Part model, mm, in its own coordinate system. Face numbers are marked on the shaded views. Coordinates: 2 decimals unless noted, no trailing zeros. Order: outer loops, then holes, each group sorted by start corner. A loop starts at its lowest first (then second) coordinate and runs counter-clockwise, first axis right, second up. Notation, with made-up numbers: (27, 83) - (74, 83) arc R22 ccw to (74, 112) - close; hole circle Ø7 at (37.25, 66). An arc over 180 degrees is marked (long way). Use a Markdown table: item, result. Add a question column.
1) Drop flat-ended pins along their axis: P1, Ø0.6, axis at x = 40.5, z = 13.5, coming from the +Y side; P2, Ø2, axis at x = -21, z = -14, coming from the -Y side; P3, Ø13, axis at x = 5.5, z = -0.5, coming from the -Y side; P4, Ø1, axis at x = -4.5, y = 16, coming from the +Z side. Give the stop position or say it passes through.
2) Saw through at D-D on y = 19. List the corners of the cut face in (x, z).
3) Saw through at A-A on x = -69. List the corners of the cut face in (y, z).
4) Two-plate mould, pull along Z, no slides. Class the marked faces 1, 2, 3 and 4: +Z half, -Z half, draft (parallel to the pull), parting line (faces both ways), or undercut.
5) Saw through at B-B on x = 26. List the corners of the cut face in (y, z), then the cut area to 3 significant figures.
6) Saw through at C-C on y = 36. List the corners of the cut face in (x, z).
7) Wall check: L1, parallel to Z at x = 46, y = 7.5; L2, parallel to Y at x = -47, z = 5; L3, parallel to Y at x = 51, z = 14. Give the ranges that are in metal, low to high. Write a range as [from, to].
```python
from build123d import *

# Parameters (mm, degrees)
BOSS_EXTRUDE1_DEPTH = 2
BOSS_EXTRUDE2_DEPTH = 26
BOSS_EXTRUDE3_START = 2
BOSS_EXTRUDE3_DEPTH = 2
CUT_EXTRUDE1_REACH  = 138.664
CUT_EXTRUDE2_DEPTH  = 137.663822213
HOLE1_D             = 1.156713631
HOLE1_DEPTH         = 2
HOLE2_D             = 7.232882037
HOLE2_DEPTH         = 2
FILLET1_R           = 2
FILLET2_R           = 4
FILLET3_R           = 6
FILLET4_R           = 7
FILLET5_R           = 9


with BuildPart() as part:
    # Sketch1 → Boss-Extrude1 (new body)
    with BuildSketch(Plane.XY.offset(-13)):
        with BuildLine():
            Line((38.589514728, 53.714517423), (38.390964743, 54.000002708))
            Line((38.390964743, 54.000002708), (37, 56.000002696))
            Line((37, 56.000002696), (-79, 56.000002696))
            Line((-79, 56.000002696), (-84.797547627, 44.113268525))
            ThreePointArc((-84.797547627, 44.113268525), (-103.30638504, 33.384611029), (-109.961112948, 13.052475123))
            ThreePointArc((-109.961112948, 13.052475123), (-114.714513302, 9.85906483), (-118.822624433, 5.869565217))
            ThreePointArc((-118.822624433, 5.869565217), (-117.511822587, -7.114760135), (-104.611841725, -5.139563921))
            Line((-104.611841725, -5.139563921), (-76.511157838, -5.139563921))
            ThreePointArc((-76.511157838, -5.139563921), (-66.310042494, -8.694638462), (-59.898757812, 0))
            Line((-59.898757812, 0), (59.520798297, 0))
            ThreePointArc((59.520798297, 0), (81.317661031, -7.891849144), (88.119135563, 14.269478708))
            Line((88.119135563, 14.269478708), (68.507754464, 49.131976199))
            Line((68.507754464, 49.131976199), (42.308532947, 53.113281503))
            Line((42.308532947, 53.113281503), (41.5, 54.000002696))
            Line((41.5, 54.000002696), (39.5, 54.000002696))
            ThreePointArc((39.5, 54.000002696), (39.14959506, 53.522905936), (38.589514728, 53.714517423))
        make_face()
    extrude(amount=-BOSS_EXTRUDE1_DEPTH)

    # Sketch2 → Boss-Extrude2 (add)
    with BuildSketch(Plane.XY.offset(-13)):
        Polygon((37, 56.000002696), (38.390964806, 54.000002752), (-79.97546515, 54.000002752), (-79, 56.000002696), align=None)
    extrude(amount=BOSS_EXTRUDE2_DEPTH)

    # Sketch3 → Boss-Extrude3 (add)
    with BuildSketch(Plane.XY.offset(13).offset(BOSS_EXTRUDE3_START)):
        with BuildLine():
            Line((39.500000002, 54.000002689), (41.499999991, 54.000002689))
            Line((41.499999991, 54.000002689), (42.308532938, 53.113281497))
            Line((42.308532938, 53.113281497), (68.507754455, 49.131976193))
            Line((68.507754455, 49.131976193), (88.119135607, 14.269478608))
            ThreePointArc((88.119135607, 14.269478608), (81.317661026, -7.891849269), (59.520798297, 0))
            Line((59.520798297, 0), (-59.898757812, 0))
            ThreePointArc((-59.898757812, 0), (-66.310042494, -8.694638462), (-76.511157838, -5.139563921))
            Line((-76.511157838, -5.139563921), (-104.611841725, -5.139563921))
            ThreePointArc((-104.611841725, -5.139563921), (-117.511822587, -7.114760135), (-118.822624433, 5.869565217))
            ThreePointArc((-118.822624433, 5.869565217), (-114.714513302, 9.85906483), (-109.961112948, 13.052475123))
            ThreePointArc((-109.961112948, 13.052475123), (-103.30638504, 33.384611029), (-84.797547627, 44.113268525))
            Line((-84.797547627, 44.113268525), (-79, 56.000002696))
            Line((-79, 56.000002696), (37, 56.000002696))
            Line((37, 56.000002696), (38.589345234, 53.714761246))
            ThreePointArc((38.589345234, 53.714761246), (39.149453375, 53.522861518), (39.500000002, 54.000002689))
        make_face()
    extrude(amount=-BOSS_EXTRUDE3_DEPTH)

    # Sketch4 → Cut-Extrude1 (cut, up to next)
    with BuildSketch(Plane(origin=(0, 0, -15), x_dir=(-1, 0, 0), z_dir=(0, 0, -1)), mode=Mode.PRIVATE) as cut_extrude1_sk1:
        with BuildLine():
            Line((-37, 14.999963704), (42, 14.999963704))
            ThreePointArc((42, 14.999963704), (48.5, 21.499963704), (42, 27.999963704))
            Line((42, 27.999963704), (-37, 27.999963704))
            ThreePointArc((-37, 27.999963704), (-43.5, 21.499963704), (-37, 14.999963704))
        make_face()
    cut_extrude1_tool1 = extrude(cut_extrude1_sk1.sketch, amount=-CUT_EXTRUDE1_REACH, mode=Mode.PRIVATE) & part.part
    add(cut_extrude1_tool1.solids().sort_by_distance((-2.5, 21.499964, -15))[0], mode=Mode.SUBTRACT)

    # Sketch5 → Cut-Extrude2 (cut, through all)
    with BuildSketch(Plane.XY.offset(15)):
        with BuildLine():
            Line((37, 27.999963704), (-42, 27.999963704))
            ThreePointArc((-42, 27.999963704), (-48.5, 21.499963704), (-42, 14.999963704))
            Line((-42, 14.999963704), (37, 14.999963704))
            ThreePointArc((37, 14.999963704), (43.5, 21.499963704), (37, 27.999963704))
        make_face()
    extrude(amount=-CUT_EXTRUDE2_DEPTH, mode=Mode.SUBTRACT)

    # Hole1
    with Locations(Plane(origin=(0, 0, 13), x_dir=(-1, 0, 0), z_dir=(0, 0, -1))):
        with Locations((-78.000162744, 0)):
            Hole(HOLE1_D / 2, depth=HOLE1_DEPTH)

    # Hole2
    with Locations(Plane.XY.offset(-13)):
        with Locations((-69, 0)):
            Hole(HOLE2_D / 2, depth=HOLE2_DEPTH)

    # Fillet1
    fillet1_edges = [part.edges().sort_by_distance(p)[0] for p in [
        (42.308532947, 53.113281503, -14),
        (42.308532938, 53.113281497, 14),
    ]]
    fillet(fillet1_edges, radius=FILLET1_R)

    # Fillet2
    fillet2_edges = [part.edges().sort_by_distance(p)[0] for p in [
        (-84.797547627, 44.113268525, -14),
        (-84.797547627, 44.113268525, 14),
    ]]
    fillet(fillet2_edges, radius=FILLET2_R)

    # Fillet3
    fillet3_edges = [part.edges().sort_by_distance(p)[0] for p in [
        (-109.961112948, 13.052475123, -14),
        (-109.961112948, 13.052475123, 14),
    ]]
    fillet(fillet3_edges, radius=FILLET3_R)

    # Fillet4
    fillet4_edges = [part.edges().sort_by_distance(p)[0] for p in [
        (-59.898757812, 0, -14),
        (-76.511157838, -5.139563921, -14),
        (-104.611841725, -5.139563921, -14),
        (-104.611841725, -5.139563921, 14),
        (-76.511157838, -5.139563921, 14),
        (-59.898757812, 0, 14),
    ]]
    fillet(fillet4_edges, radius=FILLET4_R)

    # Fillet5
    fillet5_edges = [part.edges().sort_by_distance(p)[0] for p in [
        (59.520798297, 0, -14),
        (59.520798297, 0, 14),
    ]]
    fillet(fillet5_edges, radius=FILLET5_R)


solid = part.part
```
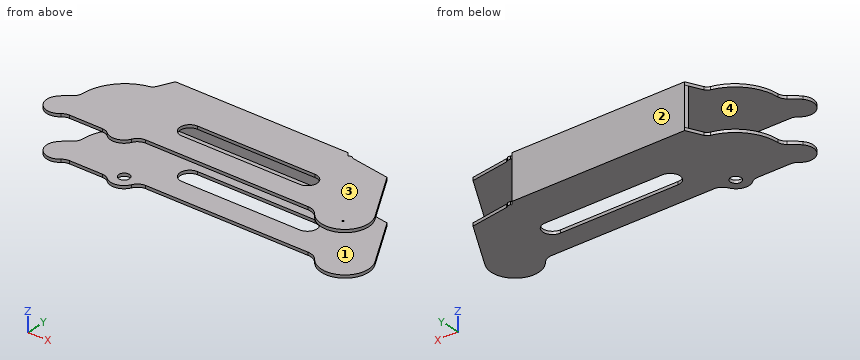
Results are:
| question | item | result |
|---|---|---|
| 1 | P1 | y = 54 |
| 1 | P2 | y = 0 |
| 1 | P3 | y = 54 |
| 1 | P4 | through |
| 2 | outline | (-109.66, -15) - (-48, -15) - (-48, -13) - (-109.66, -13) - close; (-109.66, 13) - (-48, 13) - (-48, 15) - (-109.66, 15) - close; (43, -15) - (85.46, -15) - (85.46, -13) - (43, -13) - close; (43, 13) - (85.46, 13) - (85.46, 15) - (43, 15) - close |
| 3 | outline | (-9.1, -15) - (-3.62, -15) - (-3.62, -13) - (-9.1, -13) - close; (-9.1, 13) - (54, 13) - (54, -13) - (3.62, -13) - (3.62, -15) - (56, -15) - (56, 15) - (-9.1, 15) - close |
| 4 | face 1 | undercut |
| 4 | face 2 | draft |
| 4 | face 3 | +Z half |
| 4 | face 4 | undercut |
| 5 | outline | (0, -15) - (15, -15) - (15, -13) - (0, -13) - close; (0, 13) - (15, 13) - (15, 15) - (0, 15) - close; (28, -15) - (56, -15) - (56, 15) - (28, 15) - (28, 13) - (54, 13) - (54, -13) - (28, -13) - close |
| 5 | area | 224 mm2 |
| 6 | outline | (-100.92, -15) - (75.89, -15) - (75.89, -13) - (-100.92, -13) - close; (-100.92, 13) - (75.89, 13) - (75.89, 15) - (-100.92, 15) - close |
| 7 | L1 | [-15, -13], [13, 15] |
| 7 | L2 | [54, 56] |
| 7 | L3 | [0, 51.79] |
